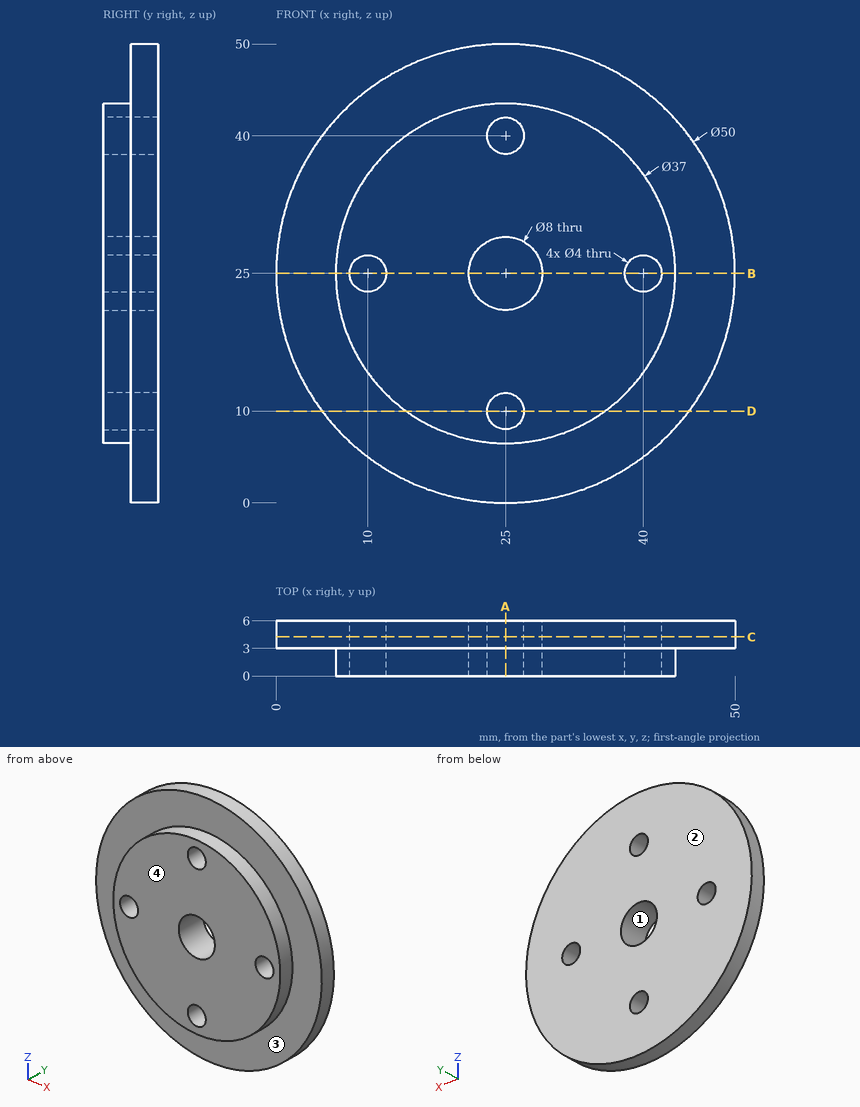
Geometry: see drawing. Coordinates: mm, zero at the bounding-box minimum. A direction names the side the tool comes from. Coordinates: 2 decimals unless noted, no trailing zeros. Loops run counter-clockwise (first coordinate to the right, second up) from the corner with the lowest first, then second, coordinate; pieces in that order, holes last.
(1) Section B-B on z = 25. Return the cut outline in (x, y).
(2) Section C-C on y = 4.25. Return the cut outline in (x, z).
(3) Set-up query: the marked faces 3 and 4. Return all of +Z, -Z, +X, -X, +Y, -Y with unobstructed straight access to the full face (end or side cutting, diameter ignored); none if empty.
(4) Material intervals for probe 1 along X at (y, z) = (4.85, 25); probe 2 along X at (y, z) = (2.95, 25); probe 3 along Z at (x, y) = (39, 2.4), sorted ascending.
(5) Section D-D on z = 10. Return the cut outline in (x, y), then the cut area to 3 significant figures.
(6) Pull-direction query (Z, two-part tool) for the marked faces 1 and 2; classes: released by +Z, released by -Z, zero draft, split by the parting line, or undercut.
(7) First-contact query: pin 1 Ø1.5 at (y, z) = (2.5, 35) entering from +X; pin 2 Ø3.5 at (x, z) = (25, 40) entering from -Y; pin 3 Ø4 at (x, z) = (10.5, 45) entering from -Y; pin 4 Ø2 at (y, z) = (1.5, 36.5) entering from -X. Flat tips, straight axial feed; report the tip coordinate or a pass-through.
(8) Section A-A on x = 25. Return the cut outline in (y, z), then the cut area to 3 significant figures.
Data:
1. outline: (0, 3) - (6.5, 3) - (6.5, 0) - (8, 0) - (8, 6) - (0, 6) - close; (12, 0) - (21, 0) - (21, 6) - (12, 6) - close; (29, 0) - (38, 0) - (38, 6) - (29, 6) - close; (42, 0) - (43.5, 0) - (43.5, 3) - (50, 3) - (50, 6) - (42, 6) - close
2. outline: circle Ø50 at (25, 25); hole circle Ø4 at (10, 25); hole circle Ø8 at (25, 25); hole circle Ø4 at (25, 10); hole circle Ø4 at (25, 40); hole circle Ø4 at (40, 25)
3. face 3: -Y
3. face 4: +Z, -Z, +X, -X, -Y
4. probe 1: x = 0 to 8, 12 to 21, 29 to 38, 42 to 50
4. probe 2: x = 6.5 to 8, 12 to 21, 29 to 38, 42 to 43.5
4. probe 3: z = 12.91 to 23.27, 26.73 to 37.09
5. outline: (5, 3) - (14.17, 3) - (14.17, 0) - (23, 0) - (23, 6) - (5, 6) - close; (27, 0) - (35.83, 0) - (35.83, 3) - (45, 3) - (45, 6) - (27, 6) - close
5. area: 161 mm2
6. face 1: undercut
6. face 2: zero draft
7. pin 1: stops at x = 48.15
7. pin 2: passes through
7. pin 3: stops at y = 3
7. pin 4: stops at x = 9.77
8. outline: (0, 6.5) - (3, 6.5) - (3, 0) - (6, 0) - (6, 8) - (0, 8) - close; (0, 12) - (6, 12) - (6, 21) - (0, 21) - close; (0, 29) - (6, 29) - (6, 38) - (0, 38) - close; (0, 42) - (6, 42) - (6, 50) - (3, 50) - (3, 43.5) - (0, 43.5) - close
8. area: 165 mm2
